Here's how the part is built. I have some questions about the finished solid (model axes, mm). Face numbers are marked on the shaded views. A direction names the side the tool comes from. Coordinates: 2 decimals unless noted, no trailing zeros. Order: outer loops, then holes, each group sorted by start corner. A loop starts at its lowest first (then second) coordinate and runs counter-clockwise, first axis right, second up. Notation, with made-up numbers: (-6, -28.75) - (31, -28.75) arc R27 cw to (31, 5.25) - close; hole circle Ø5 at (-21.5, -26). An arc over 180 degrees is marked (long way). Use one line per item in the form item = value. Start each with the question number.
from build123d import *

# Parameters (mm, degrees)
BOSS_EXTRUDE1_DEPTH = 5
SKETCH4_R           = 2
CUT_EXTRUDE1_DEPTH  = 10
SKETCH5_R           = 4
CUT_EXTRUDE2_DEPTH  = 10


with BuildPart() as part:
    # Sketch2 → Boss-Extrude1 (new body)
    with BuildSketch(Plane.XY):
        with BuildLine():
            Line((5.061398723, -21.923326458), (29.57885851, -39.211882372))
            Line((29.57885851, -39.211882372), (46.867414424, -14.694422585))
            Line((46.867414424, -14.694422585), (22.349954637, 2.594133329))
            ThreePointArc((22.349954637, 2.594133329), (0, 22.5), (-22.349954637, 2.594133329))
            Line((-22.349954637, 2.594133329), (-46.867414424, -14.694422585))
            Line((-46.867414424, -14.694422585), (-29.57885851, -39.211882372))
            Line((-29.57885851, -39.211882372), (-5.061398723, -21.923326458))
            ThreePointArc((-5.061398723, -21.923326458), (0, -22.5), (5.061398723, -21.923326458))
        make_face()
    extrude(amount=BOSS_EXTRUDE1_DEPTH)

    # Sketch4 → Cut-Extrude1 (cut)
    with BuildSketch(Plane.XY.offset(5)):
        with Locations((-39.89974514, -15.899239897)):
            Circle(SKETCH4_R)
        with Locations((-23.554771949, -4.373535954)):
            Circle(SKETCH4_R)
        with Locations((-12.029068006, -20.718509146)):
            Circle(SKETCH4_R)
        with Locations((-28.374041198, -32.244213088)):
            Circle(SKETCH4_R)
        with Locations((23.554771949, -4.373535954)):
            Circle(SKETCH4_R)
        with Locations((12.029068006, -20.718509146)):
            Circle(SKETCH4_R)
        with Locations((39.89974514, -15.899239897)):
            Circle(SKETCH4_R)
        with Locations((28.374041198, -32.244213088)):
            Circle(SKETCH4_R)
    extrude(amount=-CUT_EXTRUDE1_DEPTH, mode=Mode.SUBTRACT)

    # Sketch5 → Cut-Extrude2 (cut)
    with BuildSketch(Plane.XY.offset(5)):
        with Locations((0, 7.5)):
            Circle(SKETCH5_R)
    extrude(amount=-CUT_EXTRUDE2_DEPTH, mode=Mode.SUBTRACT)


solid = part.part
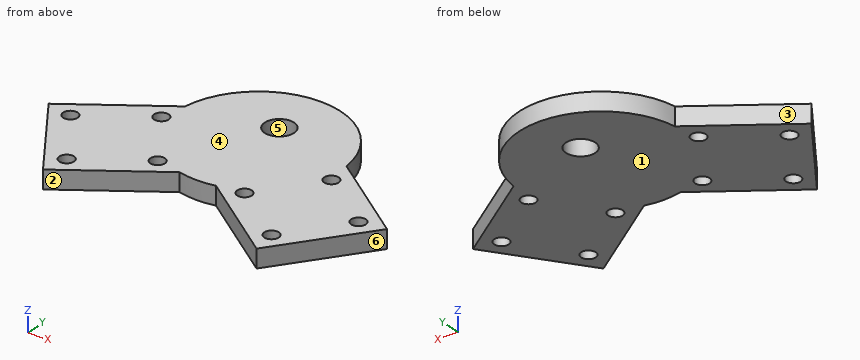
1) Suppose I cut it at D-D, the plane x = -16.5. List the corners of the cut face in (y, z) for me.
2) Suppose I cut it at B-B, the plane y = 7.5. List the corners of the cut face in (x, z) for me.
3) Suppose I cut it at A-A, the plane x = 0. List the corners of the cut face in (y, z) for me, then the cut area to 3 significant figures.
4) I need wall thicknesses on probe 1 along X at (y, z) = (-4, 1.3); probe 2 along X at (y, z) = (-5, 4.3); probe 3 along X at (y, z) = (-25, 1.6). Which ranges of each line are inside material? Lowest first, please. Write a range as [from, to].
5) If we mould it in two halves opening along Y, with no side actions, what happens to the marked faces 3, 4, 5 and 6? For each: pulls with the +Y half, pulls with the -Y half, needs draft (parallel to the pull), parting line crosses it, or undercut.
6) For pin 1 (6.5 mm diameter, centred on x = -28.37, y = -32.24, fed in from +Z); pin 2 (1 mm diameter, centred on y = -18, z = 3.5, fed in from +X); pin 3 (1.5 mm diameter, centred on x = 20.5, z = 4, fed in from -Y); pin 4 (1 mm diameter, centred on x = -13.5, z = 4.5, fed in from -Y), each with a flat end and sliding along its axis, tell me the tip position at first contact or that it passes through.
7) Suppose I cut it at C-C, the plane z = 1.2. Give the number of separate pieces and of enclosed holes in the cut face, then the cut area to 3 significant figures.
8) Which directions (+Z, -Z, +X, -X, +Y, -Y) give clear straight access to the entire face, cutting with the end or side of a thin tool? Please do the marked faces 1 and 2.
From the geometry:
q1.outline = (-29.99, 0) - (15.3, 0) - (15.3, 5) - (-29.99, 5) - close
q2.outline = (-21.21, 0) - (-4, 0) - (-4, 5) - (-21.21, 5) - close; (4, 0) - (21.21, 0) - (21.21, 5) - (4, 5) - close
q3.outline = (-22.5, 0) - (3.5, 0) - (3.5, 5) - (-22.5, 5) - close; (11.5, 0) - (22.5, 0) - (22.5, 5) - (11.5, 5) - close
q3.area = 185 mm2
q4.probe_1 = [-31.7, -25.52], [-21.59, 21.59], [25.52, 31.7]
q4.probe_2 = [-33.12, -25.45], [-21.66, 21.66], [25.45, 33.12]
q4.probe_3 = [-39.6, -9.42], [9.42, 39.6]
q5.face_3 = pulls with the +Y half
q5.face_4 = needs draft
q5.face_5 = undercut
q5.face_6 = pulls with the -Y half
q6.pin_1 = 5
q6.pin_2 = 44.89
q6.pin_3 = -33.34
q6.pin_4 = -28.23
q7.separate_pieces = 1
q7.enclosed_holes = 9
q7.area = 3,000 mm2
q8.face_1 = -Z, +X, -X, +Y, -Y
q8.face_2 = +Z, -Z, -Y
